The listing builds one solid part. Answer for the finished solid, in the listing's coordinates (mm). Face numbers are marked on the shaded views. A direction names the side the tool comes from. Round coordinates to 2 decimals unless told otherwise and drop trailing zeros. Loops run counter-clockwise (first coordinate to the right, second up) from the corner with the lowest first, then second, coordinate; pieces in that order, holes last. Notation, with made-up numbers: M -1,6 L 45,6 A27 cw 45,32 Z; hole C 76,-11.5 d1. An arc over 180 degrees is marked long. Answer as a JSON object with one key per item and string values.
```python
from build123d import *

# Parameters (mm, degrees)
F1_DEPTH  = 25.4
F2_R      = 6.35
F3_DEPTH  = 25.4
F5_DEPTH  = 25.4
F8_DEPTH  = 25.4
F10_DEPTH = 25.4


with BuildPart() as f1:
    # F0 (on Front) → F1 (new body)
    with BuildSketch(Plane.XZ):
        Polygon((0, 38.1), (0, 0), (63.5, 0), (63.5, 12.7), (19.05, 12.7), (19.05, 38.1), align=None)
    extrude(amount=F1_DEPTH)

    # F2 (on face) → F3 (cut)
    with BuildSketch(Plane.XY.offset(12.7)):
        with Locations((31.7500038045, -12.7)):
            Circle(F2_R)
        with Locations((50.8, -12.7120396)):
            Circle(F2_R)
    extrude(amount=-F3_DEPTH, mode=Mode.SUBTRACT)

    # F4 (on face) → F5 (cut)
    with BuildSketch(Plane.XY.offset(12.7)):
        with BuildLine():
            ThreePointArc((63.5, -12.7), (59.7802561211, -21.6802561211), (50.8, -25.4))
            Line((50.8, -25.4), (63.5, -25.4))
            Line((63.5, -25.4), (63.5, -12.7))
        make_face()
        with BuildLine():
            ThreePointArc((50.8, 0), (59.7802561211, -3.7197438789), (63.5, -12.7))
            Line((63.5, -12.7), (63.5, 0))
            Line((63.5, 0), (50.8, 0))
        make_face()
    extrude(amount=-F5_DEPTH, mode=Mode.SUBTRACT)

    # F7 (on face) → F8 (cut)
    with BuildSketch(Plane.YZ.offset(19.05)):
        with BuildLine():
            ThreePointArc((-19.05, 25.4), (-12.7, 19.05), (-6.35, 25.4))
            ThreePointArc((-6.35, 25.4), (-12.7, 31.75), (-19.05, 25.4))
        make_face()
        with BuildLine():
            ThreePointArc((-19.05, 25.4), (-12.7, 31.75), (-6.35, 25.4))
            Line((-6.35, 25.4), (-6.35, 38.1))
            Line((-6.35, 38.1), (-19.05, 38.1))
            Line((-19.05, 38.1), (-19.05, 25.4))
        make_face()
    extrude(amount=-F8_DEPTH, mode=Mode.SUBTRACT)

    # F9 (on face) → F10 (cut)
    with BuildSketch(Plane.YZ.offset(19.05)):
        with BuildLine():
            ThreePointArc((-25.4, 31.75), (-12.7, 36.6009683429), (0, 31.75))
            Line((0, 31.75), (0, 38.1))
            Line((0, 38.1), (-25.4, 38.1))
            Line((-25.4, 38.1), (-25.4, 31.75))
        make_face()
    extrude(amount=-F10_DEPTH, mode=Mode.SUBTRACT)


solid = f1.part
```
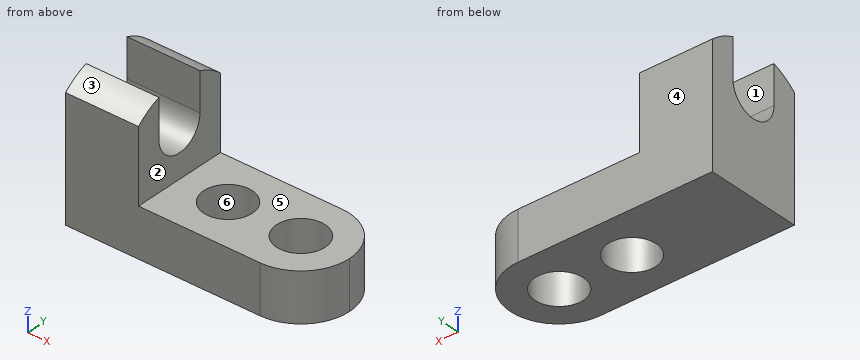
Item 1: Flat-ended cylindrical pins translate along their axes: P1, Ø1.5, axis at x = 33.5, y = -22.5, coming from the +Z side; P2, Ø12, axis at x = 9.5, y = -18, coming from the -Z side; P3, Ø2, axis at y = -18.5, z = 18, coming from the +X side; P4, Ø10, axis at x = 50.8, y = -12.71, coming from the -Z side. Find the tip coordinate at first contact, or state that the pin passes through.
Values follow:
{"P1": "z = 12.7", "P2": "z = 0", "P3": "x = 19.05", "P4": "through"}
Item 2: The part is cut by section B-B (y = -11). Give the vertices of the cut face in (x, z).
Values follow:
{"outline": "M 0,0 L 25.63,0 L 25.63,12.7 L 19.05,12.7 L 19.05,19.28 L 0,19.28 Z; M 37.87,0 L 44.69,0 L 44.69,12.7 L 37.87,12.7 Z; M 56.91,0 L 63.39,0 L 63.39,12.7 L 56.91,12.7 Z"}
Item 3: Which of the six approach directions +Z, -Z, +X, -X, +Y, -Y give full straight-line access (tool end or side, diameter ignored) to the marked faces 1, 2 and 3?
Values follow:
{"face 1": "+Z, +X, -X", "face 2": "+Z, +X, +Y, -Y", "face 3": "+Z, +X, -X, -Y"}
Item 4: The part is cut by section D-D (x = 53). Give the vertices of the cut face in (y, z), then the cut area to 3 significant figures.
Values follow:
{"outline": "M -25.21,0 L -18.67,0 L -18.67,12.7 L -25.21,12.7 Z; M -6.76,0 L -0.19,0 L -0.19,12.7 L -6.76,12.7 Z", "area": "166 mm^2"}
Item 5: Determine the mould class of the marked faces 4, 5 and 6 for opening direction Y: released by +Y, released by -Y, zero draft, split by the parting line, or undercut.
Values follow:
{"face 4": "released by +Y", "face 5": "zero draft", "face 6": "undercut"}
Item 6: The part is cut by section C-C (x = 9.5). Give the vertices of the cut face in (y, z).
Values follow:
{"outline": "M -25.4,0 L 0,0 L 0,31.75 A19.05 ccw -6.35,35.51 L -6.35,25.4 A6.35 cw -19.05,25.4 L -19.05,35.51 A19.05 ccw -25.4,31.75 Z"}
Item 7: Straight lines are drawn through the part: line 1 (Y direction, x = 15, z = 26); line 2 (Z direction, x = 56, y = -18.5); line 3 (X direction, y = -6, z = 24). For each, find the intervals that lie inside material, in ascending order.
Values follow:
{"line 1": "-25.4 to -19.05, -6.35 to 0", "line 2": "0 to 12.7", "line 3": "0 to 19.05"}
Item 8: The part is cut by section A-A (z = 32.5). Give the vertices of the cut face in (x, y), then the cut area to 3 significant figures.
Values follow:
{"outline": "M 0,-24.51 L 19.05,-24.51 L 19.05,-19.05 L 0,-19.05 Z; M 0,-6.35 L 19.05,-6.35 L 19.05,-0.89 L 0,-0.89 Z", "area": "208 mm^2"}
